CAD build for the part. Positions are in the model's coordinates, mm. A direction names the side the tool comes from. Coordinates: 2 decimals unless noted, no trailing zeros. Loops run counter-clockwise (first coordinate to the right, second up) from the corner with the lowest first, then second, coordinate; pieces in that order, holes last. Notation, with made-up numbers: (-21, 36) -> (-7, 36) arc R19 ccw to (-7, 71) -> close; hole circle Ø1 at (40, 83.25). An arc over 180 degrees is marked (long way). Write each question's results on one line, items separated by ' | '.
```python
from build123d import *

# Parameters (mm, degrees)
SKETCH1_R      = 20.125
SKETCH1_R_2    = 5.25
EXTRUDE1_DEPTH = 10


with BuildPart() as part:
    # Sketch1 → Extrude1 (new body)
    with BuildSketch(Plane.XY):
        with BuildLine():
            Line((-37.923361282, 2.412191764), (-72.084536873, -23.800600209))
            ThreePointArc((-72.084536873, -23.800600209), (-80.704195785, -28.407903885), (-90.347379744, -30))
            Line((-90.347379744, -30), (-266.026334039, -30))
            ThreePointArc((-266.026334039, -30), (-268.886721807, -32.095465966), (-267.751212763, -35.454545455))
            ThreePointArc((-267.751212763, -35.454545455), (-255.500241033, -65.45565953), (-277.670674774, -89.090909091))
            ThreePointArc((-277.670674774, -89.090909091), (-279.805574248, -92.880647284), (-275.911681822, -94.819077862))
            Line((-275.911681822, -94.819077862), (-224.773076173, -76.206147584))
            ThreePointArc((-224.773076173, -76.206147584), (-221.40563686, -75.30384494), (-217.932673306, -75))
            Line((-217.932673306, -75), (-9.777154065, -75))
            ThreePointArc((-9.777154065, -75), (-2.78855267, -73.010526422), (2.10446711, -67.638663429))
            Line((2.10446711, -67.638663429), (28.653113345, -14.247775111))
            ThreePointArc((28.653113345, -14.247775111), (13.889557824, 28.828461344), (-28.999331175, 13.529182954))
            ThreePointArc((-28.999331175, 13.529182954), (-32.791417533, 7.432910208), (-37.923361282, 2.412191764))
        make_face()
        Circle(SKETCH1_R, mode=Mode.SUBTRACT)
        with Locations((-9.777154065, -61.730521287)):
            Circle(SKETCH1_R_2, mode=Mode.SUBTRACT)
    extrude(amount=EXTRUDE1_DEPTH)


solid = part.part
```
Q1. Cut at D-D on y = -82.5. Write the cut outline in (x, z), and give its area (3 significant figures).
Results are:
outline: (-265.16, 0) -> (-242.07, 0) -> (-242.07, 10) -> (-265.16, 10) -> close | area: 231 mm^2
Q2. Wall check: L1, parallel to Y at x = -12.5, z = 8; L2, parallel to X at y = -1, z = 4; L3, parallel to Y at x = -264, z = 6.5. Give the ranges that are in metal, low to high. Write a range as from..to.
Results are:
L1: -75..-66.22, -57.24..-15.77, 15.77..29.46 | L2: -42.37..-20.1, 20.1..31.98 | L3: -90.48..-81.42, -38.58..-30
Q3. Drop flat-ended pins along their axis: pin 1 (4 mm diameter, centred on x = -186.5, z = 6, fed in from -Y); pin 2 (6 mm diameter, centred on y = -30, z = 6.5, fed in from +X); pin 3 (2 mm diameter, centred on x = -33, z = 8.5, fed in from +Y). Give the stop position or say it passes through.
Results are:
pin 1: y = -75 | pin 2: x = 22.31 | pin 3: y = 8.46
Q4. Cut at C-C on x = -126.5. Write the cut outline in (y, z).
Results are:
outline: (-75, 0) -> (-30, 0) -> (-30, 10) -> (-75, 10) -> close
Q5. Which spindle directions (+Z, -Z, +X, -X, +Y, -Y) get a long thin tool onto all of the face, cutting with end or side? Do faces 1 (the flat face through (-177, -30, 5)), 2 (the flat face through (-115, -75, 5)), 3 (the flat face through (-91, -45, 10)). Say none if no direction does.
Results are:
face 1: +Z, -Z, -X, +Y | face 2: +Z, -Z, +X, -Y | face 3: +Z, +X, -X, +Y, -Y
Q6. Cut at A-A on y = -9.5. Write the cut outline in (x, z).
Results are:
outline: (-53.45, 0) -> (-17.74, 0) -> (-17.74, 10) -> (-53.45, 10) -> close; (17.74, 0) -> (30.56, 0) -> (30.56, 10) -> (17.74, 10) -> close
Q7. Cut at B-B on z = 7.5. Write the cut outline in (x, y) (3 decimals), and give its area (3 significant figures).
Results are:
outline: (-277.671, -89.091) arc R3 ccw (long way) to (-275.912, -94.819) -> (-224.773, -76.206) arc R20 cw to (-217.933, -75) -> (-9.777, -75) arc R13.269 ccw to (2.104, -67.639) -> (28.653, -14.248) arc R32 ccw (long way) to (-28.999, 13.529) arc R30 cw to (-37.923, 2.412) -> (-72.085, -23.801) arc R30 cw to (-90.347, -30) -> (-266.026, -30) arc R3 ccw to (-267.751, -35.455) arc R30 cw to start; hole circle Ø40.25 at (0, 0); hole circle Ø10.5 at (-9.777, -61.731) | area: 15,400 mm^2
